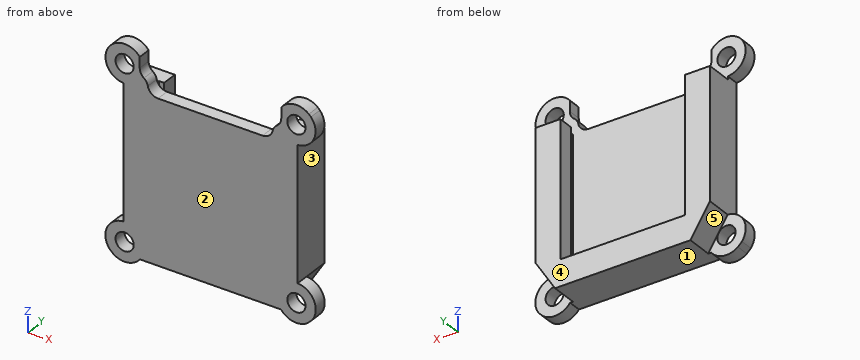
Autodesk Inventor part; units mm, degrees
ref_plane "YZ Plane" through (0, 0, 0) normal (1, 0, 0) x (0, 1, 0)
sketch "Skizze1" plane through (0, 0, 0) normal (0, 1, 0) x (-1, 0, 0)
  circle A0 centre (0, 0) radius 30
  circle A1 centre (0, 0) radius 27
  dimension "d0" = 60
  dimension "d1" = 54
extrude "Extrusion1" add sketch "Skizze1" along normal mid plane 10
sketch "Skizze5" plane through (0, 0, 0) normal (0, 1, 0) x (-1, 0, 0)
  line L0 (12.75, -14.75) -> (-12.75, -14.75)
  line L1 (-12.75, -14.75) -> (-12.75, 14.75)
  line L2 (-12.75, 14.75) -> (12.75, 14.75)
  line L3 (12.75, 14.75) -> (12.75, -14.75)
  line L4 (49.4097, 0) -> (-52.5504, 0) construction
  line L5 (0, -53.7913) -> (0, 68.1535) construction
  line L6 (-16.75, -18.75) -> (16.75, -18.75)
  line L7 (16.75, -18.75) -> (16.75, 18.75)
  line L8 (16.75, 18.75) -> (-16.75, 18.75)
  line L9 (-16.75, 18.75) -> (-16.75, -18.75)
  point P0 (0, 0)
  dimension "d33" = 29.5
  dimension "d34" = 25.5
  dimension "d35" = 4
extrude "Extrusion5" add sketch "Skizze5" along normal mid plane 2.5 contours L0 L1 L2 L3 | L9 L8 L7 L6
ref_plane "Arbeitsebene1" through (0, 0, 0) normal (0, 1, 0) x (-1, 0, 0)
chamfer "Fase1" distance 1 angle 45 2 edges at (30, 5, 0) (30, -5, 0)
sketch "Skizze2" plane through (0, 0, 0) normal (0, 1, 0) x (-1, 0, 0)
  line L0 (0, 42.2301) -> (0, -36.7007) construction
  line L1 (32.6355, 0) -> (-32.6355, 0) construction
  line L2 (16.5, 34.419) -> (16.5, -40.3324) construction
  line L3 (-16.5, 35.4304) -> (-16.5, -34.8157) construction
  line L4 (23.5881, 16.5) -> (-32.0387, 16.5) construction
  line L5 (23.5881, -16.5) -> (-39.8541, -16.5) construction
  circle A0 centre (16.5, -16.5) radius 1.75
  circle A1 centre (16.5, 16.5) radius 1.75
  circle A2 centre (-16.5, 16.5) radius 1.75
  circle A3 centre (-16.5, -16.5) radius 1.75
  circle A4 centre (-16.5, 16.5) radius 3.6749
  circle A5 centre (-16.5, -16.5) radius 3.7161
  circle A6 centre (16.5, -16.5) radius 3.7
  circle A7 centre (16.5, 16.5) radius 3.6747
  point P0 (0, 0)
  dimension "d8" = 33
  dimension "d9" = 33
  dimension "d10" = 3.5
  dimension "d11" = 3.5
  dimension "d12" = 3.5
  dimension "d13" = 3.5
extrude "Extrusion2" add sketch "Skizze2" along normal mid plane 2.5
ref_plane "Arbeitsebene2" through (0, 0, -30.5) normal (0, 0, 1) x (1, 0, 0)
extrude "Extrusion6" cut sketch "Skizze2" against normal mid plane 3 contours A0 | A1 | A2 | A3
sketch "Skizze12" plane through (0, 5, 0) normal (0, 1, 0) x (1, 0, 0)
  circle A0 centre (0, 0) radius 27
  circle A1 centre (0, 0) radius 31.5802
extrude "Extrusion13" cut sketch "Skizze12" against normal blind 10
sketch "Skizze13" plane through (0, 1.25, 0) normal (0, 1, 0) x (1, 0, 0)
  line L0 (-13.5947, -18.75) -> (13.5944, -18.75)
  line L1 (-13.5947, -18.75) -> (13.5944, -18.75)
  line L2 (13.5944, -18.75) -> (13.5944, -14.75)
  line L3 (13.5944, -14.75) -> (-13.5947, -14.75)
  line L4 (-13.5947, -14.75) -> (-13.5947, -18.75)
  point P0 (0, 0)
  dimension "d58" = 4
extrude "Extrusion14" cut sketch "Skizze13" against normal blind 3
sketch "Skizze14" plane through (0, 1.25, 0) normal (0, 1, 0) x (1, 0, 0)
  line L0 (-13, -12.25) -> (13, -12.25)
  line L1 (13, -12.25) -> (13, 13.75)
  line L2 (13, 13.75) -> (-13, 13.75)
  line L3 (-13, 13.75) -> (-13, -12.25)
  line L4 (0, -43.7267) -> (0, 49.5069) construction
  line L5 (-24.7381, 0) -> (29.5694, 0) construction
  line L6 (13.5425, 18.75) -> (-13.5627, 18.75) construction
  line L7 (-13, -12.25) -> (-16.75, -12.25)
  line L8 (-16.75, 12.8084) -> (-16.75, -12.8338)
  line L9 (-16.75, -12.25) -> (-16.75, 12.815)
  line L10 (-16.75, 12.815) -> (-13.0013, 18.75)
  line L11 (13, -12.25) -> (16.75, -12.25)
  line L12 (16.75, -12.8336) -> (16.75, 12.7924)
  arc A0 (16.75, 12.7924) -> (19.551, 18.6215) centre (16.5, 16.5) ccw
  line L13 (16.75, -12.25) -> (16.75, 12.7924)
  line L14 (16.75, 12.7924) -> (13.0013, 18.75)
  line L15 (13.0013, 18.75) -> (-13.0013, 18.75)
  point P0 (0, 0)
  dimension "d62" = 26
  dimension "d63" = 26
  dimension "d64" = 5
extrude "Extrusion15" add sketch "Skizze14" along normal blind 5 contours L7 L8 L9 L10 L15 L14 L12 L11 L1 L2 L3
sketch "Skizze15" plane through (0, 6.25, 0) normal (0, 1, 0) x (1, 0, 0)
  line L0 (-13, 13.75) -> (-13, -12.25)
  line L1 (13, 13.75) -> (-13, 13.75)
  line L2 (-13, -12.25) -> (-12, -12.25)
  line L3 (-12, -12.25) -> (-12, 13.75)
  line L4 (-12, 13.75) -> (-13, 13.75)
  line L5 (-13, 13.75) -> (-13, -12.25)
  line L6 (13, -12.25) -> (16.75, -12.25)
  line L7 (13, -12.25) -> (12, -12.25)
  line L8 (12, -12.25) -> (12, 13.75)
  line L9 (12, 13.75) -> (13, 13.75)
  line L10 (13, 13.75) -> (13, -12.25)
  point P0 (0, 0)
  dimension "d67" = 1
  dimension "d68" = 1
extrude "Extrusion16" add sketch "Skizze15" against normal blind 3
sketch "Skizze16" plane through (0, 1.25, 0) normal (0, 1, 0) x (1, 0, 0)
  line L0 (12, -12.25) -> (12, 13.75)
  line L1 (12, -12.25) -> (-12.0731, -12.25)
  line L2 (-12.0731, -12.25) -> (-12.0731, -16.1057)
  line L3 (-12.0731, -16.1057) -> (12, -16.1057)
  line L4 (12, -16.1057) -> (12, -12.25)
  point P0 (0, 0)
extrude "Extrusion17" cut sketch "Skizze16" against normal blind 10
fillet "Rundung5" radius 2 6 edges at (-13.5947, 0, 14.75) (-12.0731, 0, 14.75) (-12.0731, 0, 12.25) (12, 0, 12.25) (12, 0, 14.75) (13.5944, 0, 14.75)
properties part number "_3D-Druck"
Work out the finished part from the listing and answer in its coordinate system (mm). Face numbers are marked on the shaded views. A direction names the side the tool comes from. Give positions to 0.01 mm unless a question says otherwise; leave off trailing zeros. Loops run counter-clockwise (first coordinate to the right, second up) from the corner with the lowest first, then second, coordinate; pieces in that order, holes last. Notation, with made-up numbers: (56, 82) -> (113, 82) arc R29 cw to (113, 110) -> close; hole circle Ø6 at (23.5, -35.5). An arc over 180 degrees is marked (long way). Use a Markdown table: item, result. Add a question column.
1. For the marked faces 4 and 5, determine the directions among +Z, -Z, +X, -X, +Y, -Y from which every point of the face is accessible in a straight line to the end or side of a thin tool.
2. Section D-D on x = -6 is taken. Determine the outline of the cut face in (y, z), and give its area (4 significant figures).
3. Flat-ended cylindrical pins translate along their axes: pin 1 Ø4 at (x, y) = (13.5, 2) entering from -Z (3 decimals); pin 2 Ø2.5 at (y, z) = (5, 5) entering from -X; pin 3 Ø2 at (y, z) = (1.5, 14) entering from -X. Find the tip coordinate at first contact, or state that the pin passes through.
4. Determine the mould class of the marked faces 1, 2 and 3 for opening direction Z: released by +Z, released by -Z, zero draft, split by the parting line, or undercut.
5. Find the intervals of material crossed by probe 1 along X at (y, z) = (-0.5, -16.5); probe 2 along Z at (x, y) = (-16.5, 0.2); probe 3 along X at (y, z) = (-0.6, 16.5), in increasing order.
6. Section C-C on z = 5 is taken. Determine the outline of the cut face in (x, y), and give its area (3 significant figures).
7. Section B-B on y = 0 is taken. Determine the outline of the cut face in (x, z).
8. Section A-A on z = -16.5 is taken. Determine the outline of the cut face in (x, y).
Results below:
| question | item | result |
|---|---|---|
| 1 | face 4 | +Z, -Z, +X, -X, +Y |
| 1 | face 5 | -Z, -X, +Y |
| 2 | outline | (-1.25, -18.75) -> (6.25, -18.75) -> (6.25, -13.75) -> (1.25, -13.75) -> (1.25, 12.25) -> (-1.25, 12.25) -> close |
| 2 | area | 102.5 mm^2 |
| 3 | pin 1 | stops at z = -20.035 |
| 3 | pin 2 | stops at x = -16.75 |
| 3 | pin 3 | stops at x = -19.84 |
| 4 | face 1 | released by -Z |
| 4 | face 2 | zero draft |
| 4 | face 3 | undercut |
| 5 | probe 1 | x = -20.2 to -18.25, -14.75 to 14.75, 18.25 to 20.22 |
| 5 | probe 2 | z = -20.2 to -18.25, -14.75 to 14.75, 18.25 to 20.17 |
| 5 | probe 3 | x = -20.17 to -18.25, -14.75 to -13.59, 13.58 to 14.75, 18.25 to 20.17 |
| 6 | outline | (-16.75, -1.25) -> (16.75, -1.25) -> (16.75, 6.25) -> (12, 6.25) -> (12, 3.25) -> (13, 3.25) -> (13, 1.25) -> (-13, 1.25) -> (-13, 3.25) -> (-12, 3.25) -> (-12, 6.25) -> (-16.75, 6.25) -> close |
| 6 | area | 127 mm^2 |
| 7 | outline | (-19.47, -18.7) arc R27 ccw to (-18.7, -19.47) arc R3.7 ccw to (-13.56, -18.75) -> (13.54, -18.75) arc R3.72 ccw to (18.62, -19.55) arc R27 ccw to (19.55, -18.62) arc R3.72 ccw to (16.75, -12.79) -> (16.75, 12.83) arc R3.67 ccw to (19.29, 18.89) arc R27 ccw to (18.89, 19.29) arc R3.67 ccw to (13.59, 18.75) -> (13.59, 16.71) arc R2 cw to (12.76, 15.08) arc R2 ccw to (11.96, 13.85) arc R2 cw to (10, 12.25) -> (-10.07, 12.25) arc R2 cw to (-12.04, 13.87) arc R2 ccw to (-12.8, 15.09) arc R2 cw to (-13.59, 16.69) -> (-13.59, 18.75) arc R3.67 ccw to (-18.89, 19.29) arc R27 ccw to (-19.29, 18.89) arc R3.67 ccw to (-16.75, 12.83) -> (-16.75, -12.81) arc R3.7 ccw to start; hole circle Ø3.5 at (-16.5, -16.5); hole circle Ø3.5 at (-16.5, 16.5); hole circle Ø3.5 at (16.5, -16.5); hole circle Ø3.5 at (16.5, 16.5) |
| 8 | outline | (-20.2, -1.25) -> (-18.25, -1.25) -> (-18.25, 1.25) -> (-20.2, 1.25) -> close; (-14.75, -1.25) -> (14.75, -1.25) -> (14.75, 1.25) -> (14.42, 1.25) -> (14.42, 6.25) -> (-14.42, 6.25) -> (-14.42, 1.25) -> (-14.75, 1.25) -> close; (18.25, -1.25) -> (20.22, -1.25) -> (20.22, 1.25) -> (18.25, 1.25) -> close |
